from build123d import *

# Parameters (mm, degrees)
SKETCH1_R           = 12
BOSS_EXTRUDE1_DEPTH = 2
BOSS_EXTRUDE2_DEPTH = 1
SKETCH3_R           = 10
BOSS_EXTRUDE3_DEPTH = 5
SKETCH4_R           = 6
BOSS_EXTRUDE4_DEPTH = 5
SCALE1_SCALE        = 2


with BuildPart() as part:
    # Sketch1 → Boss-Extrude1 (new body)
    with BuildSketch(Plane(origin=(0, 0, 0), x_dir=(1, 0, 0), z_dir=(0, 1, 0))):
        Circle(SKETCH1_R)
    extrude(amount=BOSS_EXTRUDE1_DEPTH)

    # Sketch2 → Boss-Extrude2 (add, symmetric)
    with BuildSketch(Plane(origin=(0, 0, 0), x_dir=(0, 0, -1), z_dir=(1, 0, 0))):
        with BuildLine():
            Line((-11.75, 2), (-11.75, 15))
            ThreePointArc((-11.75, 15), (0, 26.75), (11.75, 15))
            Line((11.75, 15), (11.75, 2))
            Line((11.75, 2), (-11.75, 2))
        make_face()
    extrude(amount=BOSS_EXTRUDE2_DEPTH, both=True)

    # Sketch3 → Boss-Extrude3 (add)
    with BuildSketch(Plane.XZ):
        Circle(SKETCH3_R)
    extrude(amount=BOSS_EXTRUDE3_DEPTH)

    # Sketch4 → Boss-Extrude4 (add, symmetric)
    with BuildSketch(Plane(origin=(0, 0, 0), x_dir=(0, 0, -1), z_dir=(1, 0, 0))):
        with Locations((0, 15)):
            Circle(SKETCH4_R)
    extrude(amount=BOSS_EXTRUDE4_DEPTH, both=True)


with BuildPart() as part_1:
    # Scale1: scaled about (0, 5.516721754, 0)
    add(part.part.scale(SCALE1_SCALE).moved(Location((0, -5.516721754, 0))))


solid = part_1.part
Check sheet for the modelled part. Datum: model origin and axes. Units: mm. A direction names the side the tool comes from. Round coordinates to 2 decimals unless told otherwise and drop trailing zeros. Order: outer loops, then holes, each group sorted by start corner. A loop starts at its lowest first (then second) coordinate and runs counter-clockwise, first axis right, second up.
Q1. Set-up check for faces 1 (the face through (6.06, 12.77, 2.6)), 2 (the face through (-5.94, 12.77, 2.6)), 3 (the face through (10, 25, 0)), 4 (the face through (-5, -5.517, -20)), 5 (the face through (0, 11, 23.5)): record each of +Z, -Z, +X, -X, +Y, -Y from which the full face is reachable in a straight line by a thin tool's end or side.
Filled sheet:
face 1: +X
face 2: -X
face 3: +Z, -Z, +X, +Y
face 4: -Y
face 5: +Z, +X, -X, +Y
Q2. Scan lines: L1, parallel to Y at x = 15, z = 12; L2, parallel to X at y = 27.5, z = -16; L3, parallel to X at y = 15, z = 6. Record each from-to range of solid material in increasing order.
Filled sheet:
L1: y = -15.52 to -1.52
L2: x = -2 to 2
L3: x = -10 to 10
Q3. Cross-section at B-B, the plane x = -3. Enter the section's corners in (y, z), plus the area to 3 significant figures.
Filled sheet:
outline: (-15.52, -19.77) - (-5.52, -19.77) - (-5.52, -23.81) - (-1.52, -23.81) - (-1.52, 23.81) - (-5.52, 23.81) - (-5.52, 19.77) - (-15.52, 19.77) - close; circle Ø24 at (24.48, 0)
area: 1,040 mm2
Q4. Depth check by flat-ended pin: P1, Ø3, axis at x = 1, y = 6, coming from the +Z side; P2, Ø5, axis at y = -5.5, z = -10, coming from the -X side; P3, Ø1.5, axis at y = 15, z = 0.5, coming from the +X side. Enter the tip coordinate at first touch or a pass-through.
Filled sheet:
P1: stops at z = 23.5
P2: stops at x = -22.8
P3: stops at x = 10
Q5. Cross-section at A-A, the plane z = 0. Enter the section's corners in (x, y), plus the area to 3 significant figures.
Filled sheet:
outline: (-24, -5.52) - (-20, -5.52) - (-20, -15.52) - (20, -15.52) - (20, -5.52) - (24, -5.52) - (24, -1.52) - (2, -1.52) - (2, 12.48) - (10, 12.48) - (10, 36.48) - (2, 36.48) - (2, 47.98) - (-2, 47.98) - (-2, 36.48) - (-10, 36.48) - (-10, 12.48) - (-2, 12.48) - (-2, -1.52) - (-24, -1.52) - close
area: 1,170 mm2
Q6. Draft check along Y on faces 6 (the face through (0.028, 47.978, 0.517)), 7 (the face through (0, 12, -23.5)), 8 (the face through (5, -1.517, 0)). Enter one of: pulls with the +Y half, pulls with the -Y half, needs draft (parallel to the pull), parting line crosses it, or undercut.
Filled sheet:
face 6: pulls with the +Y half
face 7: needs draft
face 8: undercut
Q7. Cross-section at D-D, the plane z = -9.5. Enter the section's corners in (x, y).
Filled sheet:
outline: (-22.04, -5.52) - (-17.6, -5.52) - (-17.6, -15.52) - (17.6, -15.52) - (17.6, -5.52) - (22.04, -5.52) - (22.04, -1.52) - (2, -1.52) - (2, 17.15) - (10, 17.15) - (10, 31.81) - (2, 31.81) - (2, 45.98) - (-2, 45.98) - (-2, 31.81) - (-10, 31.81) - (-10, 17.15) - (-2, 17.15) - (-2, -1.52) - (-22.04, -1.52) - close
Q8. Cross-section at C-C, the plane y = -7. Enter the section's corners in (x, z).
Filled sheet:
outline: circle Ø40 at (0, 0)
